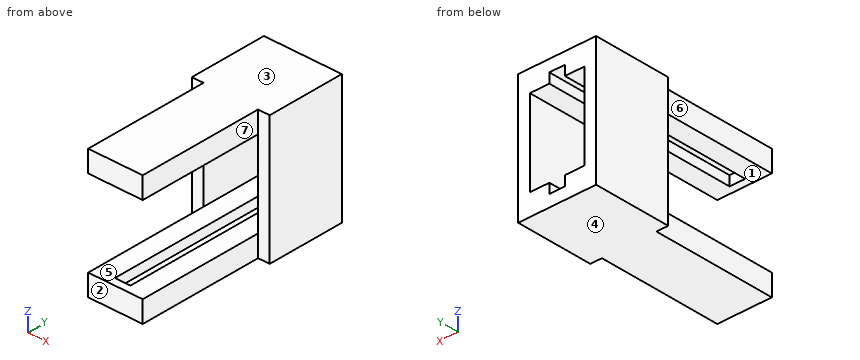
Autodesk Inventor part; units mm, degrees
ref_plane "YZ Plane" through (0, 0, 0) normal (1, 0, 0) x (0, 1, 0)
ref_plane "XZ Plane" through (0, 0, 0) normal (0, 1, 0) x (-1, 0, 0)
ref_plane "XY Plane" through (0, 0, 0) normal (0, 0, 1) x (1, 0, 0)
sketch "Sketch1" plane through (0, 0, 0) normal (0, 1, 0) x (-1, 0, 0)
  line L0 (1, 6.75) -> (3.5, 6.75)
  line L1 (3.5, 6.75) -> (3.5, 5.5)
  line L2 (3.5, 5.5) -> (1, 5.5)
  line L3 (1, 5.5) -> (1, 6.75)
  line L4 (1, 6.75) -> (3.5, 5.5) construction
  line L5 (3.5, 6.75) -> (1, 5.5) construction
  line L6 (1, -5.5) -> (3.5, -5.5)
  line L7 (3.5, -5.5) -> (3.5, -6.75)
  line L8 (3.5, -6.75) -> (1, -6.75)
  line L9 (1, -6.75) -> (1, -5.5)
  line L10 (1, -5.5) -> (3.5, -6.75) construction
  line L11 (3.5, -5.5) -> (1, -6.75) construction
  line L12 (-1, 6.75) -> (-3.5, 6.75)
  line L13 (-3.5, 6.75) -> (-3.5, 5.5)
  line L14 (-3.5, 5.5) -> (-1, 5.5)
  line L15 (-1, 5.5) -> (-1, 6.75)
  line L16 (-1, 6.75) -> (-3.5, 5.5) construction
  line L17 (-3.5, 6.75) -> (-1, 5.5) construction
  line L18 (-1, -5.5) -> (-3.5, -5.5)
  line L19 (-3.5, -5.5) -> (-3.5, -6.75)
  line L20 (-3.5, -6.75) -> (-1, -6.75)
  line L21 (-1, -6.75) -> (-1, -5.5)
  line L22 (-1, -5.5) -> (-3.5, -6.75) construction
  line L23 (-3.5, -5.5) -> (-1, -6.75) construction
  line L24 (3.5, -6.75) -> (-3.5, -6.75)
  line L25 (-3.5, -6.75) -> (-3.5, -8.25)
  line L26 (-3.5, -8.25) -> (3.5, -8.25)
  line L27 (3.5, -8.25) -> (3.5, -6.75)
  line L28 (3.5, 6.75) -> (-3.5, 6.75)
  line L29 (-3.5, 6.75) -> (-3.5, 8.25)
  line L30 (-3.5, 8.25) -> (3.5, 8.25)
  line L31 (3.5, 8.25) -> (3.5, 6.75)
  point P0 (0, 0)
  point P1 (2.25, 6.125)
  point P2 (2.25, -6.125)
  point P3 (-2.25, 6.125)
  point P4 (-2.25, -6.125)
  point P5 (2.25, 6.125)
  point P6 (2.25, -6.125)
  point P7 (-2.25, 6.125)
  point P8 (-2.25, -6.125)
  point P9 (2.25, -6.125)
  point P10 (-2.25, -6.125)
  point P11 (2.25, 6.125)
  point P12 (-2.25, 6.125)
  dimension "d0" = 2
  dimension "d1" = 11
  dimension "d2" = 5.5
  dimension "d3" = 1
  dimension "d5" = 2.5
  dimension "d6" = 13.5
  dimension "d7" = 1.5
extrude "Extrusion1" add sketch "Sketch1" against normal blind 25
sketch "Sketch2" plane through (0, 0, 0) normal (0, 1, 0) x (1, 0, 0)
  line L0 (3.5, 5.5) -> (3.5, 8.25)
  line L1 (3.5, 8.25) -> (5, 8.25)
  line L2 (5, 8.25) -> (5, -8.25)
  line L3 (5, -8.25) -> (3.5, -8.25)
  line L4 (3.5, -8.25) -> (3.5, 8.25)
  line L5 (-3.5, 8.25) -> (-3.5, 5.5)
  line L6 (-3.5, 8.25) -> (-5, 8.25)
  line L7 (-5, 8.25) -> (-5, -8.25)
  line L8 (-5, -8.25) -> (-3.5, -8.25)
  line L9 (-3.5, -8.25) -> (-3.5, 8.25)
  point P0 (0, 0)
  dimension "d10" = 1.5
extrude "Extrusion2" add sketch "Sketch2" against normal blind 10
sketch "Sketch3" plane through (0, -25, 0) normal (0, -1, 0) x (1, 0, 0)
  line L0 (-3.5, 5.5) -> (-1, 5.5)
  line L1 (3.5, 5.5) -> (3.5, 8.25)
  line L2 (-3.5, 5.5) -> (3.5, 5.5)
  line L3 (3.5, 5.5) -> (3.5, 8.25)
  line L4 (3.5, 8.25) -> (-3.5, 8.25)
  line L5 (-3.5, 8.25) -> (-3.5, 5.5)
  line L6 (3.5, -5.5) -> (1, -5.5)
  line L7 (-3.5, -5.5) -> (-3.5, -8.25)
  line L8 (3.5, -5.5) -> (-3.5, -5.5)
  line L9 (-3.5, -5.5) -> (-3.5, -8.25)
  line L10 (-3.5, -8.25) -> (3.5, -8.25)
  line L11 (3.5, -8.25) -> (3.5, -5.5)
  point P0 (0, 0)
extrude "Extrusion3" add sketch "Sketch3" along normal blind 1
properties part number "Colorimeter_Mounting-Tool"
For this review, take the finished solid that the model builds, in its own axes (mm). Face numbers are marked on the shaded views. A direction names the side the tool comes from. Coordinates: 2 decimals unless noted, no trailing zeros. Order: outer loops, then holes, each group sorted by start corner. A loop starts at its lowest first (then second) coordinate and runs counter-clockwise, first axis right, second up. Notation, with made-up numbers: (4.5, -2) -> (43.5, -2) arc R24 ccw to (43.5, 24) -> close; hole circle Ø9 at (84.5, -7.75). An arc over 180 degrees is marked (long way). Use CSV: the item, a comma, the result in double quotes. Start each with the question number.
Item 1: We need section D-D, the plane x = 0.5. Give the boundary of the cut face in (y, z).
Item 2: Insertion check: pin 1 (1.6 mm diameter, centred on x = 4.5, z = 3.5, fed in from -Y); pin 2 (1.4 mm diameter, centred on y = -19.5, z = -7.5, fed in from +X); pin 3 (1 mm diameter, centred on x = 0, z = 6, fed in from +Y). Each pin has a flat end and moves straight along its axis. Give the tip position at first contact, or say it passes through.
Item 3: Wall thickness on probe 1 along Z at (x, y) = (0.5, -24.5); probe 2 along Z at (x, y) = (1.5, -6.25); probe 3 along X at (y, z) = (-19.25, 6): over which ranges is each line inside the solid? List them lowest first.
Item 4: We need section A-A, the plane x = -2.25. Give the boundary of the cut face in (y, z), then the cut area to 3 significant figures.
Item 5: We need section B-B, the plane y = -11. Give the boundary of the cut face in (x, z).
Item 6: For the marked faces 5, 6 and 7, list the 3-axis set-ups (+Z, -Z, +X, -X, +Y, -Y) from which the entire face can be reached by the end or side of a thin tool; tool diameter is ignored.
Item 7: Draft analysis for pull direction Z (two halves, no side actions). For the marked faces 1, 2, 3 and 4, state which applies: pulls with the +Z half, pulls with the -Z half, needs draft (parallel to the pull), parting line crosses it, or undercut.
Item 8: We need section C-C, the plane z = 2.25. Give the boundary of the cut face in (x, y), then the cut area to 3 significant figures.
Derived:
1,outline,"(-26, -8.25) -> (0, -8.25) -> (0, -6.75) -> (-25, -6.75) -> (-25, -5.5) -> (-26, -5.5) -> close; (-26, 5.5) -> (-25, 5.5) -> (-25, 6.75) -> (0, 6.75) -> (0, 8.25) -> (-26, 8.25) -> close"
2,pin 1,"stops at y = -10"
2,pin 2,"stops at x = 3.5"
2,pin 3,"stops at y = -25"
3,probe 1,"z = -8.25 to -6.75, 6.75 to 8.25"
3,probe 2,"z = -8.25 to -5.5, 5.5 to 8.25"
3,probe 3,"x = -3.5 to -1, 1 to 3.5"
4,outline,"(-26, -8.25) -> (0, -8.25) -> (0, -5.5) -> (-26, -5.5) -> close; (-26, 5.5) -> (0, 5.5) -> (0, 8.25) -> (-26, 8.25) -> close"
4,area,"143 mm^2"
5,outline,"(-3.5, -8.25) -> (3.5, -8.25) -> (3.5, -5.5) -> (1, -5.5) -> (1, -6.75) -> (-1, -6.75) -> (-1, -5.5) -> (-3.5, -5.5) -> close; (-3.5, 5.5) -> (-1, 5.5) -> (-1, 6.75) -> (1, 6.75) -> (1, 5.5) -> (3.5, 5.5) -> (3.5, 8.25) -> (-3.5, 8.25) -> close"
6,face 5,"+Y, -Y"
6,face 6,"+Z, -Z, -X, -Y"
6,face 7,"+Z, -Z, +X, -Y"
7,face 1,"undercut"
7,face 2,"needs draft"
7,face 3,"pulls with the +Z half"
7,face 4,"pulls with the -Z half"
8,outline,"(-5, -10) -> (-3.5, -10) -> (-3.5, 0) -> (-5, 0) -> close; (3.5, -10) -> (5, -10) -> (5, 0) -> (3.5, 0) -> close"
8,area,"30.0 mm^2"
